Build history of the part. All positions in model axes, mm. A direction names the side the tool comes from. Round coordinates to 2 decimals unless told otherwise and drop trailing zeros. Write each loop counter-clockwise with the first axis right and the second up, starting at its lowest first coordinate (ties: lowest second). Pieces come first, ordered by that corner, then holes. Notation, with made-up numbers: (-17, 60.25) - (-2, 60.25) arc R26 cw to (-2, 97.25) - close; hole circle Ø10 at (87.5, 29.5). An arc over 180 degrees is marked (long way). Answer as a JSON object with one key per item and string values. Group by question number.
Item 1: Slice it at A-A, the plane z = 11.5. List the corners of the cut face in (x, y), then the cut area to 3 significant figures.
Item 2: Slice it at C-C, the plane y = 7. List the corners of the cut face in (x, z), then the cut area to 3 significant figures.
Item 3: Which spindle directions (+Z, -Z, +X, -X, +Y, -Y) get a long thin tool onto all of the face, cutting with end or side? Do faces 1 (the flat face through (8, 8, 9.843)), 2 (the flat face through (7, 8, 7.343)), 3 (the flat face through (14.8, -2, 8)), 4 (the flat face through (8, 2, 0.8)), 5 (the flat face through (5, -5, 8)). Say none if no direction does.
Item 4: Slice it at D-D, the plane z = 7.8. List the corners of the cut face in (x, y), then the cut area to 3 significant figures.
Item 5: Flat gauge pins, fed straight in: pin 1 (1.5 mm diameter, centred on y = -3, z = 8.5, fed in from -X); pin 2 (2 mm diameter, centred on x = 10.5, z = 7, fed in from +Y); pin 3 (1.6 mm diameter, centred on y = 8, z = 6.5, fed in from -X); pin 4 (0.8 mm diameter, centred on x = 9, y = 7.5, fed in from +Z). Where does each tip first touch, or does it go through?
Item 6: Slice it at B-B, the plane x = 7.8. List the corners of the cut face in (y, z), then the cut area to 3 significant figures.
Item 7: Probe line 1 (Z direction, x = 1.5, y = -0.75); line 2 (Y direction, x = 5.75, z = 6). List the from-to ranges inside material, lowest first. Write a range as from..to.
Autodesk Fusion 360 part; units mm, degrees
sketch "Sketch1" plane through (0, 0, 0) normal (0, 1, 0) x (1, 0, 0)
  line L0 (0, 0) -> (15.6, 0)
  line L1 (15.6, 0) -> (15.6, -15.6)
  line L2 (15.6, -15.6) -> (0, -15.6)
  line L3 (0, -15.6) -> (0, 0)
  dimension "d1" = 15.6
  dimension "d2" = 15.6
extrude "Extrude1" add sketch "Sketch1" along normal blind 1
sketch "Sketch4" plane through (0, 0, 0) normal (0, -1, 0) x (1, 0, 0)
  line L0 (15.6, 15.6) -> (0, 15.6)
  line L1 (0, 15.6) -> (0, 0)
  line L2 (0, 0) -> (15.6, 0)
  line L3 (15.6, 0) -> (15.6, 15.6)
  line L4 (0.8, 14.8) -> (14.8, 14.8)
  line L5 (14.8, 14.8) -> (14.8, 0.8)
  line L6 (14.8, 0.8) -> (0.8, 0.8)
  line L7 (0.8, 0.8) -> (0.8, 14.8)
  dimension "d7" = 0.8
  dimension "d8" = 0.8
  dimension "d9" = 0.8
  dimension "d10" = 0.8
extrude "Extrude2" add sketch "Sketch4" along normal blind 5 contours L4 L5 L6 L7
sketch "Sketch5" plane through (0, 1, 0) normal (0, 1, 0) x (-1, 0, 0)
  line L0 (0, 15.6) -> (-15.6, 15.6)
  line L1 (-15.6, 15.6) -> (-15.6, 0)
  line L2 (-15.6, 0) -> (0, 0)
  line L3 (0, 0) -> (0, 15.6)
  line L4 (-0.8, 0.8) -> (-14.8, 0.8)
  line L5 (-14.8, 0.8) -> (-14.8, 14.8)
  line L6 (-14.8, 14.8) -> (-0.8, 14.8)
  line L7 (-0.8, 14.8) -> (-0.8, 0.8)
  dimension "d13" = 0.8
  dimension "d14" = 0.8
  dimension "d15" = 0.8
  dimension "d16" = 0.8
extrude "Extrude3" add sketch "Sketch5" along normal blind 5.6 contours L4 L5 L6 L7
fillet "Fillet1" radius 3 4 edges at (7.8, 6.6, 0.8) (14.8, 6.6, 7.8) (7.8, 6.6, 14.8) (0.8, 6.6, 7.8)
sketch "Sketch6" plane through (0, 6.6, 0) normal (0, 1, 0) x (-1, 0, 0)
  line L0 (-3.8, 11.8) -> (-11.8, 11.8)
  line L1 (-11.8, 11.8) -> (-11.8, 3.8)
  line L2 (-11.8, 3.8) -> (-3.8, 3.8)
  line L3 (-3.8, 3.8) -> (-3.8, 11.8)
  line L4 (-8.3063, 7.3427) -> (-8.3063, 5.8427)
  line L5 (-8.3063, 7.3427) -> (-9.8063, 7.3427)
  line L6 (-8.3063, 5.8427) -> (-7.3063, 5.8427)
  line L7 (-7.3063, 5.8427) -> (-7.3063, 7.3427)
  line L8 (-7.3063, 7.3427) -> (-5.8063, 7.3427)
  line L9 (-5.8063, 7.3427) -> (-5.8063, 8.3427)
  line L10 (-5.8063, 8.3427) -> (-7.3063, 8.3427)
  line L11 (-7.3063, 8.3427) -> (-7.3063, 9.8427)
  line L12 (-7.3063, 9.8427) -> (-8.3063, 9.8427)
  line L13 (-8.3063, 9.8427) -> (-8.3063, 8.3427)
  line L14 (-8.3063, 8.3427) -> (-9.8063, 8.3427)
  line L15 (-9.8063, 8.3427) -> (-9.8063, 7.3427)
extrude "Extrude4" add sketch "Sketch6" along normal blind 3.6 contours L4 L5 L6 L7 L8 L9 L10 L11 L12 L13 L14 L15
sketch "Sketch7" plane through (0, -5, 0) normal (0, -1, 0) x (1, 0, 0)
  line L0 (0.8, 0.8) -> (14.8, 0.8)
  line L1 (14.8, 0.8) -> (14.8, 14.8)
  line L2 (14.8, 14.8) -> (0.8, 14.8)
  line L3 (0.8, 14.8) -> (0.8, 0.8)
  circle A0 centre (7.8, 7.8) radius 2.5
extrude "Extrude5" add sketch "Sketch7" along normal blind 3.3 contours A0
chamfer "Chamfer1" distance 1 angle 45 1 edges at (5.4692, -8.3, 6.896)
Geometry says:
{
 "1": {"outline": "(0, 0) - (0.8, 0) - (0.8, -5) - (14.8, -5) - (14.8, 0) - (15.6, 0) - (15.6, 1) - (14.8, 1) - (14.8, 3.6) arc R3 ccw to (11.8, 6.6) - (3.8, 6.6) arc R3 ccw to (0.8, 3.6) - (0.8, 1) - (0, 1) - close", "area": "160 mm^2"},
 "2": {"outline": "(5.81, 7.34) - (7.31, 7.34) - (7.31, 5.84) - (8.31, 5.84) - (8.31, 7.34) - (9.81, 7.34) - (9.81, 8.34) - (8.31, 8.34) - (8.31, 9.84) - (7.31, 9.84) - (7.31, 8.34) - (5.81, 8.34) - close", "area": "7.00 mm^2"},
 "3": {"face 1": "+Z, +X, -X, +Y", "face 2": "-Z, -X, +Y", "face 3": "+Z, -Z, +X, -Y", "face 4": "-Z, +X, -X, +Y", "face 5": "-Y"},
 "4": {"outline": "(0, 0) - (0.8, 0) - (0.8, -5) - (5.3, -5) - (5.3, -7.3) - (6.3, -8.3) - (9.3, -8.3) - (10.3, -7.3) - (10.3, -5) - (14.8, -5) - (14.8, 0) - (15.6, 0) - (15.6, 1) - (14.8, 1) - (14.8, 3.6) arc R3 ccw to (11.8, 6.6) - (9.81, 6.6) - (9.81, 10.2) - (5.81, 10.2) - (5.81, 6.6) - (3.8, 6.6) arc R3 ccw to (0.8, 3.6) - (0.8, 1) - (0, 1) - close", "area": "190 mm^2"},
 "5": {"pin 1": "stops at x = 0.8", "pin 2": "stops at y = 10.2", "pin 3": "stops at x = 7.31", "pin 4": "stops at z = 8.34"},
 "6": {"outline": "(-8.3, 6.3) - (-7.3, 5.3) - (-5, 5.3) - (-5, 0.8) - (0, 0.8) - (0, 0) - (1, 0) - (1, 0.8) - (3.6, 0.8) arc R3 ccw to (6.6, 3.8) - (6.6, 5.84) - (10.2, 5.84) - (10.2, 9.84) - (6.6, 9.84) - (6.6, 11.8) arc R3 ccw to (3.6, 14.8) - (1, 14.8) - (1, 15.6) - (0, 15.6) - (0, 14.8) - (-5, 14.8) - (-5, 10.3) - (-7.3, 10.3) - (-8.3, 9.3) - close", "area": "190 mm^2"},
 "7": {"line 1": "z = 0.8..14.8", "line 2": "y = -5..6.6"}
}
